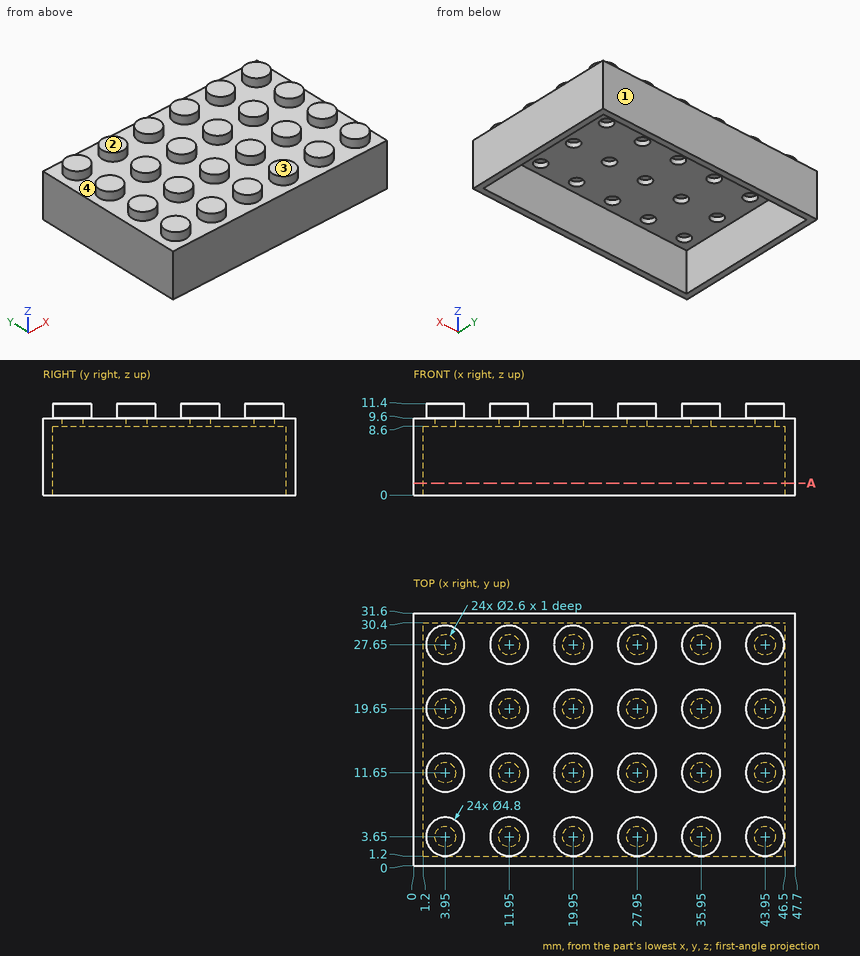
Input: dimensioned drawing with shaded views. Units: mm. Origin: part minimum x, y, z. A direction names the side the tool comes from. Round coordinates to 2 decimals unless told otherwise and drop trailing zeros. Order: outer loops, then holes, each group sorted by start corner. A loop starts at its lowest first (then second) coordinate and runs counter-clockwise, first axis right, second up. Notation, with made-up numbers: (32.5, 51) -> (49.5, 51) arc R19 cw to (49.5, 72) -> close; hole circle Ø1 at (6, -27). An arc over 180 degrees is marked (long way). Put each result on its own line as item: value. Start each with the question number.
Q1. Line query: probe 1 along Y at (x, z) = (19.95, 8.95); probe 2 along X at (y, z) = (27, 6.75); probe 3 along Y at (x, z) = (38, 5). Output: solid intervals per line, ascending.
Q2. Pull-direction query (Z, two-part tool) for the marked faces 1 and 2; classes: +Z half, -Z half, draft (parallel to the pull), parting line (faces both ways), or undercut.
Q3. Section A-A on z = 1.5. Return the cut outline in (x, y).
Q4. First-contact query: pin 1 (3 mm diameter, centred on x = 27.5, y = 4, fed in from -Z); pin 2 (0.8 mm diameter, centred on x = 4, y = 27.5, fed in from -Z). Flat tips, straight axial feed; report the tip coordinate or a pass-through.
Q5. Reachability of the marked faces 3 and 4 from +Z, -Z, +X, -X, +Y, -Y: full face, straight path, thin tool, end or side. Return the list, or none.
Ans:
1. probe 1: y = 0 to 2.35, 4.95 to 10.35, 12.95 to 18.35, 20.95 to 26.35, 28.95 to 31.6
1. probe 2: x = 0 to 1.2, 46.5 to 47.7
1. probe 3: y = 0 to 1.2, 30.4 to 31.6
2. face 1: draft
2. face 2: +Z half
3. outline: (0, 0) -> (47.7, 0) -> (47.7, 31.6) -> (0, 31.6) -> close; hole (1.2, 1.2) -> (46.5, 1.2) -> (46.5, 30.4) -> (1.2, 30.4) -> close
4. pin 1: stops at z = 8.6
4. pin 2: stops at z = 9.6
5. face 3: +Z, +X, -X, +Y, -Y
5. face 4: +Z
